```python
from build123d import *

# Parameters (mm, degrees)
FILLET1_R          = 1.5
SKETCH3_R          = 10
CUT_EXTRUDE1_DEPTH = 136.5
FILLET2_R          = 3
FILLET3_R          = 3


with BuildPart() as part:
    # Sketch1 → Revolve1 (revolve)
    with BuildSketch(Plane.XY, mode=Mode.PRIVATE) as revolve1_sk:
        Polygon((0, 0), (300, 0), (300, 15), (271.419940235, 15), (271.419940235, 12), (268.089940235, 12), (268.089940235, 18), (46.35, 18), (46.35, 15), (40, 15), (40, 30), (0, 30), align=None)
    revolve(revolve1_sk.sketch.rotate(Axis((0, 0, 0), (1, 0, 0)), 90), axis=Axis((0, 0, 0), (1, 0, 0)))

    # Fillet1
    fillet1_edges = [part.edges().sort_by_distance(p)[0] for p in [
        (0, 0, -30),
    ]]
    fillet(fillet1_edges, radius=FILLET1_R)

    # Sketch3 → Cut-Extrude1 (cut, symmetric)
    with BuildSketch(Plane.XY):
        with Locations((20, 0)):
            Circle(SKETCH3_R)
    extrude(amount=CUT_EXTRUDE1_DEPTH, both=True, mode=Mode.SUBTRACT)

    # Fillet2
    fillet2_edges = [part.edges().sort_by_distance(p)[0] for p in [
        (40, 0, -15),
    ]]
    fillet(fillet2_edges, radius=FILLET2_R)

    # Fillet3
    fillet3_edges = [part.edges().sort_by_distance(p)[0] for p in [
        (40, 0, -30),
    ]]
    fillet(fillet3_edges, radius=FILLET3_R)


solid = part.part
```
Build history of the part. All positions in model axes, mm. A direction names the side the tool comes from. Round coordinates to 2 decimals unless told otherwise and drop trailing zeros. Write each loop counter-clockwise with the first axis right and the second up, starting at its lowest first coordinate (ties: lowest second). Pieces come first, ordered by that corner, then holes.
1) Drill centre lines: probe 1 along X at (y, z) = (0, 7); probe 2 along X at (y, z) = (0, -17); probe 3 along X at (y, z) = (-11, 13.5). Where is each one in solid material? Low to high.
2) Band-saw the part on B-B, the plane z = 0. List the corners of the cut face in (x, y), and give its area (3 significant figures).
3) Mould opens along X. For faces 4 (the flat face through (0, 0, 0)), 5 (the cylindrical face through (285.51, -12.65, 8.06)), 6 (the flat face through (268.09, 12, -4)) say: +X half, -X half, draft (parallel to the pull), parting line (faces both ways), or undercut.
4) Band-saw the part on D-D, the plane x = 20. List the corners of the cut face in (y, z).
5) 3-axis set-ups, long thin cutter, end or side, ignore diameter. For faces 1 (the cylindrical face through (44.65, -12.65, 8.06)), 2 (the cylindrical face through (19.002, 11.49, 27.712)), 3 (the flat face through (40, 6, -18)): which of +Z, -Z, +X, -X, +Y, -Y reach the whole face in a straight line?
6) Band-saw the part on C-C, the plane x = 213.5. List the corners of the cut face in (y, z).
7) Pin check, flat tips, straight feed: pin 1 (1.5 mm diameter, centred on x = 158.5, z = 5.5, fed in from +Y); pin 2 (5 mm diameter, centred on x = 92.5, y = 17.5, fed in from +Z); pin 3 (12 mm diameter, centred on x = 147, y = -15.5, fed in from -Z). Stop position of each tip, or through.
Ans:
1. probe 1: x = 0 to 10, 30 to 300
1. probe 2: x = 0 to 10, 30 to 40.17, 46.35 to 268.09
1. probe 3: x = 0 to 40.06, 46.35 to 268.09
2. outline: (0, -28.5) arc R1.5 ccw to (1.5, -30) - (37, -30) arc R3 ccw to (40, -27) - (40, -18) arc R3 cw to (43, -15) - (46.35, -15) - (46.35, -18) - (268.09, -18) - (268.09, -12) - (271.42, -12) - (271.42, -15) - (300, -15) - (300, 15) - (271.42, 15) - (271.42, 12) - (268.09, 12) - (268.09, 18) - (46.35, 18) - (46.35, 15) - (43, 15) arc R3 cw to (40, 18) - (40, 27) arc R3 ccw to (37, 30) - (1.5, 30) arc R1.5 ccw to (0, 28.5) - close; hole circle Ø20 at (20, 0)
2. area: 11,200 mm2
3. face 4: -X half
3. face 5: draft
3. face 6: undercut
4. outline: (-10, -28.28) - (-10, 28.28) arc R30 ccw to start; (10, -28.28) arc R30 ccw to (10, 28.28) - close
5. face 1: none
5. face 2: +X, -X
5. face 3: +X
6. outline: circle Ø36 at (0, 0)
7. pin 1: stops at y = 17.36
7. pin 2: stops at z = 9.95
7. pin 3: stops at z = -15.29
